CAD build for the part. Positions are in the model's coordinates, mm. A direction names the side the tool comes from. Coordinates: 2 decimals unless noted, no trailing zeros. Order: outer loops, then holes, each group sorted by start corner. A loop starts at its lowest first (then second) coordinate and runs counter-clockwise, first axis right, second up.
from build123d import *

# Parameters (mm, degrees)
CUT_EXTRUDE1_DEPTH      = 7
SKETCH3_W               = 26.933594661
SKETCH3_H               = 5.726695828
CUT_EXTRUDE2_DEPTH      = 7.1
CUT_EXTRUDE2_DEPTH_BACK = 7.1


with BuildPart() as part:
    # Sketch1 → Revolve1 (revolve)
    with BuildSketch(Plane(origin=(0, 0, 0), x_dir=(0, 0, -1), z_dir=(1, 0, 0))):
        with BuildLine():
            Line((19.186178752, 5.078211692), (19.186178752, 6.1))
            Line((19.186178752, 6.1), (20.186178752, 6.1))
            Line((20.186178752, 6.1), (20.186178752, 5.8))
            ThreePointArc((20.186178752, 5.8), (21.211305018, 3.325126266), (23.686178752, 2.3))
            Line((23.686178752, 2.3), (41.207308429, 2.3))
            Line((41.207308429, 2.3), (41.207308429, 3.9))
            Line((41.207308429, 3.9), (42.707308429, 3.9))
            Line((42.707308429, 3.9), (42.707308429, 2.3))
            Line((42.707308429, 2.3), (54.469152884, 2.3))
            Line((54.469152884, 2.3), (54.469152884, 4.719165839))
            Line((54.469152884, 4.719165839), (57.819152884, 4.719165839))
            Line((57.819152884, 4.719165839), (57.819152884, 2.3))
            Line((57.819152884, 2.3), (59.757795324, 2.3))
            Line((59.757795324, 2.3), (59.757795324, 1.3))
            Line((59.757795324, 1.3), (23.73491848, 1.3))
            ThreePointArc((23.73491848, 1.3), (22.154791951, 1.676988608), (20.915059537, 2.72674277))
            Line((20.915059537, 2.72674277), (19.186178752, 5.078211692))
        make_face()
    revolve(axis=Axis((0, 0, 0), (0, 0, -1)))

    # Sketch2 → Cut-Extrude1 (cut)
    with BuildSketch(Plane.XY.offset(-19.186178752)):
        Polygon((2, 6), (2, 0.524681536), (7.756224258, 0.524681536), (7.708002274, 5.9580813), align=None)
    extrude(amount=-CUT_EXTRUDE1_DEPTH, mode=Mode.SUBTRACT)

    # Sketch3 → Cut-Extrude2 (cut, two sides)
    with BuildSketch(Plane(origin=(0, 0, 0), x_dir=(0, 0, -1), z_dir=(1, 0, 0))) as cut_extrude2_sk:
        with Locations((31.133671125, 5.163347914)):
            Rectangle(SKETCH3_W, SKETCH3_H)
    extrude(amount=CUT_EXTRUDE2_DEPTH, mode=Mode.SUBTRACT)
    extrude(cut_extrude2_sk.sketch, amount=-CUT_EXTRUDE2_DEPTH_BACK, mode=Mode.SUBTRACT)


solid = part.part
1) Pin check, flat tips, straight feed: P1, Ø5, axis at x = 1, y = -0.5, coming from the -Z side; P2, Ø1.5, axis at y = -2.5, z = -38.5, coming from the +X side; P3, Ø1.5, axis at x = 1, z = -52, coming from the -Y side; P4, Ø0.9, axis at y = 1.5, z = -24, coming from the +X side. Stop position of each tip, or through.
2) Which spindle directions (+Z, -Z, +X, -X, +Y, -Y) get a long thin tool onto all of the face, cutting with end or side? Do faces 5 (the cylindrical face through (-4.187, 2.178, -56.168)), 6 (the cylindrical face through (-1.4, -1.825, -32.569)), 7 (the flat face through (-1.2, 2.3, -21.3)), 8 (the cylindrical face through (1.29, -0.17, -41.49)). Say none if no direction does.
3) Drill centre lines: probe 1 along Z at (x, y) = (3, 1.5); probe 2 along Z at (x, y) = (3.75, 0); probe 3 along X at (y, z) = (0, -50.5). Where is each one in solid material? Low to high.
4) Two-plate mould, pull along X, no slides. Class faces 1 (the flat face through (-2, -5, -19.186)), 2 (the flat face through (2, 1, -23)), 3 (the cylindrical face through (-1.4, -1.825, -48.671)), 4 (the conical face through (-1.05, -2.67, -20.81)): released by +X, released by -X, zero draft, split by the parting line, or undercut.
5) Slice it at C-C (y = -3.25). Give the number of separate pieces and of enclosed holes in the cut face, plus the area to 3 significant figures.
6) Slice it at B-B (z = -30). List the corners of the cut face in (x, y), plus the area to 3 significant figures.
Worked out:
1. P1: stops at z = -59.76
1. P2: stops at x = 1.49
1. P3: stops at y = -2.29
1. P4: stops at x = 2
2. face 5: -Z
2. face 6: none
2. face 7: +Z, +X, -X, +Y
2. face 8: +Z, -Z
3. probe 1: z = -57.82 to -54.47, -42.71 to -41.21
3. probe 2: z = -57.82 to -54.47, -42.71 to -41.21, -20.85 to -20.16
3. probe 3: x = -2.3 to -1.3, 1.3 to 2.3
4. face 1: zero draft
4. face 2: released by +X
4. face 3: split by the parting line
4. face 4: undercut
5. separate pieces: 3
5. enclosed holes: 0
5. area: 38.0 mm2
6. outline: circle Ø4.6 at (0, 0); hole circle Ø2.6 at (0, 0)
6. area: 11.3 mm2
